Geometry: final body of the model. Coordinates: model frame, mm. Face numbers are marked on the shaded views. A direction names the side the tool comes from. Give positions to 0.01 mm unless a question says otherwise; leave off trailing zeros. Write each loop counter-clockwise with the first axis right and the second up, starting at its lowest first coordinate (ties: lowest second). Pieces come first, ordered by that corner, then holes. Notation, with made-up numbers: (-26.75, 53) -> (-21.75, 53) arc R11 cw to (-21.75, 66) -> close; hole circle Ø8 at (72.25, 63). An arc over 180 degrees is marked (long way). Answer as a JSON object with one key per item and string values.
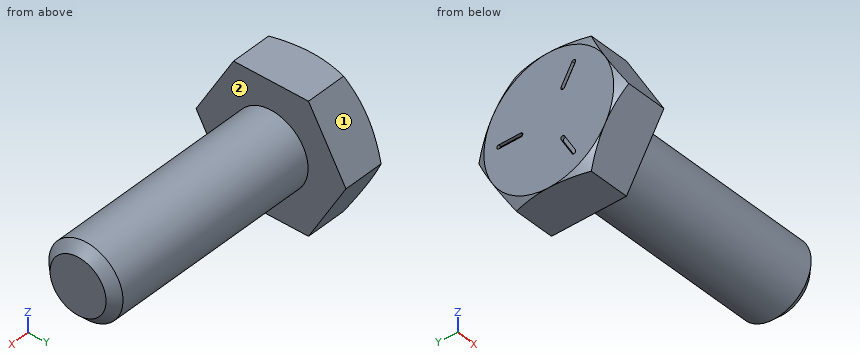
from build123d import *

# Parameters (mm, degrees)
SKETCH5_R           = 3.175
BOSS_EXTRUDE3_DEPTH = 19.05
CHAMFER1_SIZE       = 0.77724
BOSS_EXTRUDE4_DEPTH = 3.96875
SKETCH8_OUTSIDE_W   = 102.036
SKETCH8_OUTSIDE_H   = 103.756
SKETCH8_OUTSIDE_R   = 5.55625
CUT_EXTRUDE3_DEPTH  = 24.01875
CUT_EXTRUDE3_TAPER  = 60
CUT_EXTRUDE4_DEPTH  = 0.254
CIRPATTERN1_COUNT   = 3


with BuildPart() as part:
    # Sketch5 → Boss-Extrude3 (new body)
    with BuildSketch(Plane(origin=(11.509375, 0, 0), x_dir=(0, 0, -1), z_dir=(1, 0, 0))):
        Circle(SKETCH5_R)
    extrude(amount=-BOSS_EXTRUDE3_DEPTH)

    # Chamfer1
    chamfer1_edges = [part.edges().sort_by_distance(p)[0] for p in [
        (11.509375, 0, 3.175),
    ]]
    chamfer(chamfer1_edges, length=CHAMFER1_SIZE)

    # Sketch6 → Boss-Extrude4 (add)
    with BuildSketch(Plane.ZY.offset(7.540625)):
        Polygon((5.55625, 3.207902433), (0, 6.415804866), (-5.55625, 3.207902433), (-5.55625, -3.207902433), (0, -6.415804866), (5.55625, -3.207902433), align=None)
    extrude(amount=BOSS_EXTRUDE4_DEPTH)

    # Sketch8 outside → Cut-Extrude3 (cut, through all)
    with BuildSketch(Plane.ZY.offset(11.509375)):
        Rectangle(SKETCH8_OUTSIDE_W, SKETCH8_OUTSIDE_H)
        Circle(SKETCH8_OUTSIDE_R, mode=Mode.SUBTRACT)
    extrude(amount=-CUT_EXTRUDE3_DEPTH, taper=CUT_EXTRUDE3_TAPER, mode=Mode.SUBTRACT)

    # Sketch12 → Cut-Extrude4 (cut)
    with BuildSketch(Plane.ZY.offset(11.509375)):
        with BuildLine():
            Line((0.1666875, 4.2783125), (0.1666875, 2.3891875))
            ThreePointArc((0.1666875, 2.3891875), (0, 2.2225), (-0.1666875, 2.3891875))
            Line((-0.1666875, 2.3891875), (-0.1666875, 4.2783125))
            ThreePointArc((-0.1666875, 4.2783125), (0, 4.445), (0.1666875, 4.2783125))
        make_face()
    cut_extrude4 = extrude(amount=-CUT_EXTRUDE4_DEPTH, mode=Mode.SUBTRACT)

    # CirPattern1: Cut-Extrude4 ×3 about axis
    cirpattern1_axis = Axis((0, 0, 0), (1, 0, 0))
    for i in range(1, CIRPATTERN1_COUNT):
        add(cut_extrude4.rotate(cirpattern1_axis, i * 360 / CIRPATTERN1_COUNT), mode=Mode.SUBTRACT)


solid = part.part
Q1. Material intervals for L1, parallel to X at y = 4.75, z = -2.5; L2, parallel to X at y = -2, z = 3.25; L3, parallel to Y at x = -9.5, z = 1.5, sorted ascending. Write a range as from..to.
Values:
{"L1": "-11.51..-7.54", "L2": "-11.26..-7.54", "L3": "-5.55..5.55"}
Q2. First-contact query: P1, Ø6, axis at x = -2.5, y = 2, coming from the +Z side (3 decimals); P2, Ø4, axis at x = 5.5, z = -0.5, coming from the +Y side (3 decimals); P3, Ø3, axis at x = -7, z = 1.5, coming from the +Y side. Flat tips, straight axial feed; report the tip coordinate or a pass-through.
Values:
{"P1": "z = 3.175", "P2": "y = 3.175", "P3": "y = 6.36"}
Q3. Set-up query: the marked faces 1 and 2. Return all of +Z, -Z, +X, -X, +Y, -Y with unobstructed straight access to the full face (end or side cutting, diameter ignored); none if empty.
Values:
{"face 1": "+Z, +X, -X, +Y", "face 2": "+X"}
Q4. Cut plane A-A (x = 6.25). Return the cut outline in (y, z) (3 decimals).
Values:
{"outline": "circle Ø6.35 at (0, 0)"}
